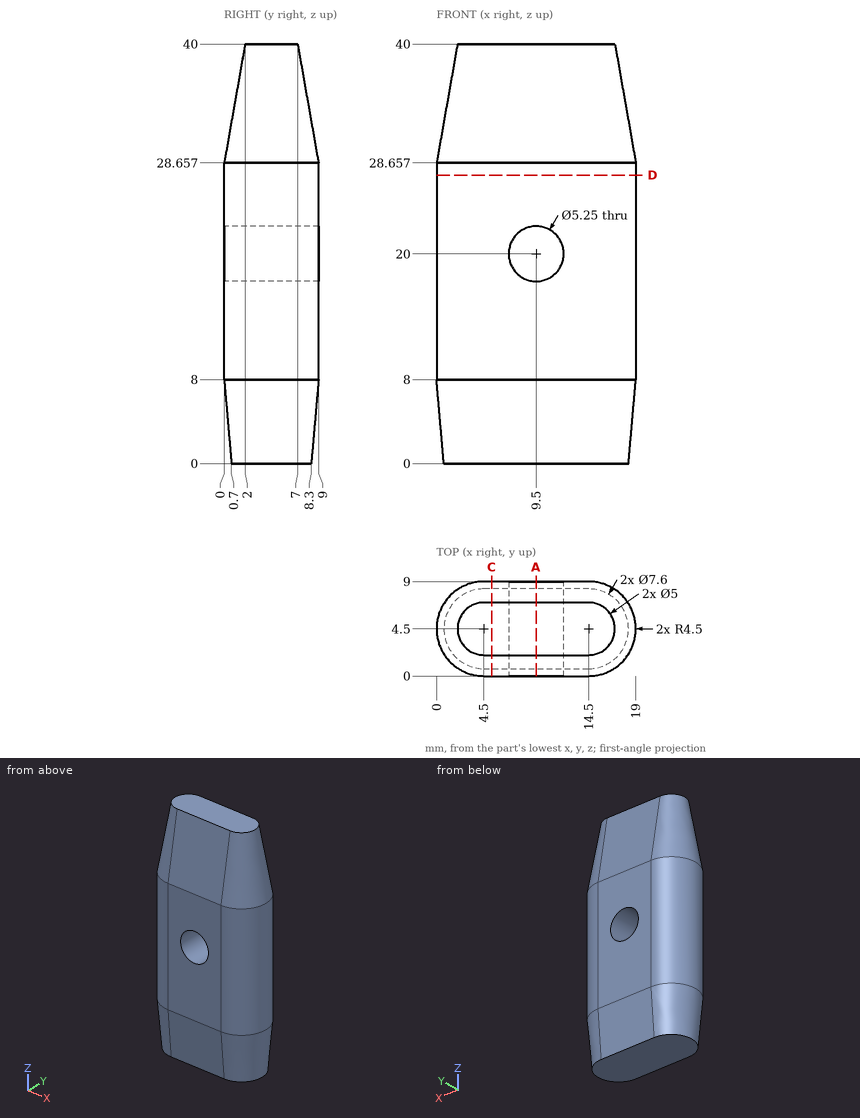
Job drawing, mm, ordinate dimensions from the low corner. One solid piece. Give positions to 0.01 mm unless a question says otherwise; leave off trailing zeros. Loops run counter-clockwise (first coordinate to the right, second up) from the corner with the lowest first, then second, coordinate; pieces in that order, holes last. Notation, with made-up numbers: M 1.25,10.25 L 13.25,10.25 A19 ccw 13.25,21.25 Z; hole C -39,18 d7. An arc over 180 degrees is marked long. Use one line per item in the form item = value.
Item 1: Flat gauge pin, fed straight in: pin 1 Ø1 at (y, z) = (3, 17) entering from -X. Where does the tip first touch, or does it go through?
Filled in:
pin_1 = 0.11
Item 2: Slice it at D-D on z = 27.5. List the corners of the cut face in (x, y), and give its area (3 significant figures).
Filled in:
outline = M 4.5,0 L 14.5,0 A4.5 ccw 14.5,9 L 4.5,9 A4.5 ccw Z
area = 154 mm^2
Item 3: Drill centre lines: L1, parallel to Z at x = 9.5, y = 6.25 (1 decimal); L2, parallel to X at y = 8.25, z = 19 (1 decimal); L3, parallel to X at y = 4.25, z = 38. Where is each one in solid material? Low to high.
Filled in:
L1 = 0 to 17.4, 22.6 to 40
L2 = 2 to 7.1, 11.9 to 17
L3 = 1.66 to 17.34
Item 4: Slice it at C-C on x = 5.25. List the corners of the cut face in (y, z).
Filled in:
outline = M 0,8 L 0.7,0 L 8.3,0 L 9,8 L 9,28.66 L 7,40 L 2,40 L 0,28.66 Z
Item 5: Slice it at A-A on x = 9.5. List the corners of the cut face in (y, z) (1 decimal).
Filled in:
outline = M 0,8 L 0.7,0 L 8.3,0 L 9,8 L 9,17.4 L 0,17.4 Z; M 0,22.6 L 9,22.6 L 9,28.7 L 7,40 L 2,40 L 0,28.7 Z
